Could you check a few things on this drawing? It's one solid part, dimensions in mm from its lowest x, y, z. A direction names the side the tool comes from. Coordinates: 2 decimals unless noted, no trailing zeros. Write each loop counter-clockwise with the first axis right and the second up, starting at its lowest first coordinate (ties: lowest second). Pieces come first, ordered by that corner, then holes. Notation, with made-up numbers: (45.25, 85.5) - (64.25, 85.5) arc R16 cw to (64.25, 93.5) - close; hole circle Ø7 at (56, -31.75). An arc over 180 degrees is marked (long way). Use one line per item in the form item = value. Start each with the question number.
(1) If we section it at B-B on y = 29.5: Please give me the cut outline in (x, z), then the cut area to 3 significant figures.
(2) If we section it at D-D on z = 19.25: Please give me the cut outline in (x, y).
(3) If we section it at A-A on x = 4: Please give me the cut outline in (y, z) (1 decimal).
(4) If I drill on probe 1 along Z at (x, y) = (14.5, 1); probe 2 along X at (y, z) = (13, 15.5) (1 decimal); probe 3 along X at (y, z) = (10, 20.25) (1 decimal), over which ranges is the centre line in solid material (lowest first)? Write a range as from..to.
(5) If we section it at C-C on z = 5: Please give me the cut outline in (x, y), then the cut area to 3 significant figures.
(6) For pin 1 Ø5 at (x, z) = (12, 14.5) entering from +Y; pin 2 Ø4 at (y, z) = (25.5, 5.5) entering from -X; pin 3 Ø12 at (y, z) = (9.5, 5) entering from -X; pin 4 Ø1.5 at (y, z) = (27, 3.5) entering from -X, each with a flat end and sliding along its axis, tell me the tip position at first contact or that it passes through.
(7) Thinking about a two-plate mould opening in Z: for the marked faces 3, 4 and 5, which applies, pulls with the +Z half, pulls with the -Z half, needs draft (parallel to the pull), parting line crosses it, or undercut?
(8) On a 3-axis mill with a long thin cutter (end or side, diameter ignored), from which of +Z, -Z, +X, -X, +Y, -Y can I reach the whole of each face in a straight line? I mean the marked faces 1 and 2. Say none if no direction works.
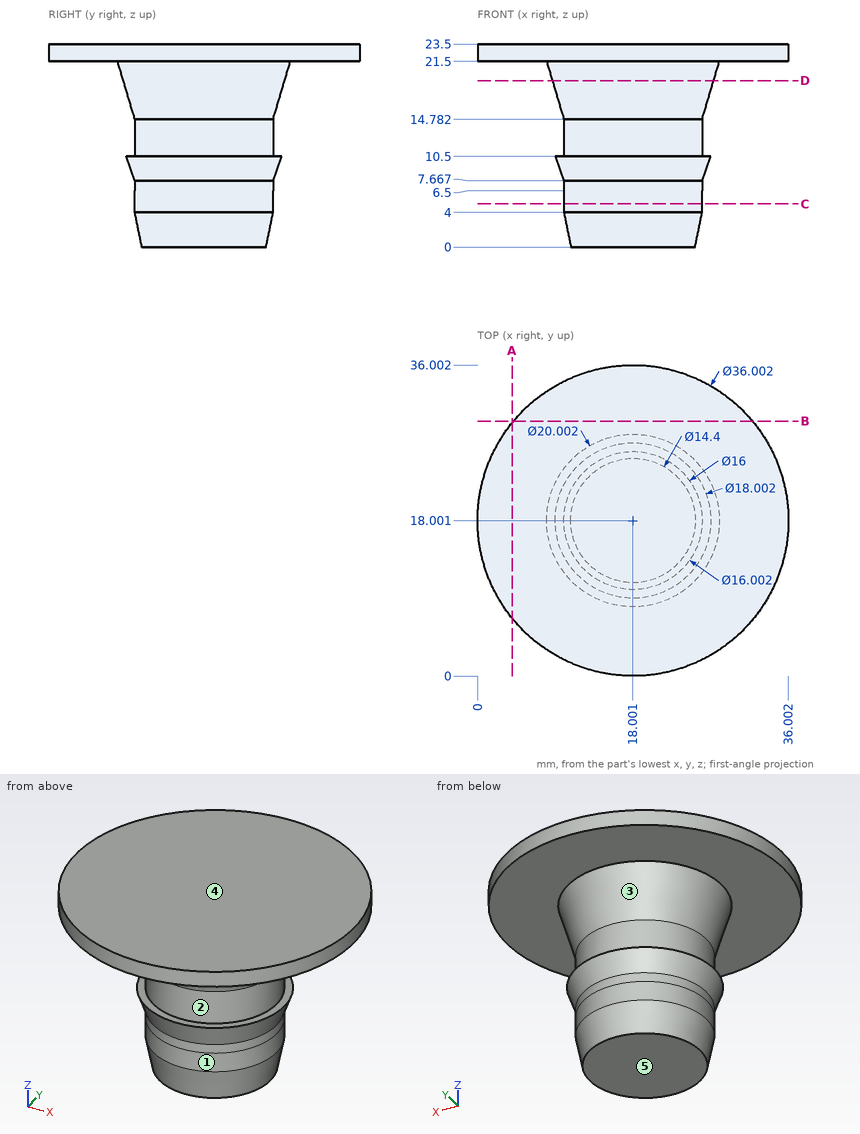
Reported:
q1.outline = (4.15, 21.5) - (31.85, 21.5) - (31.85, 23.5) - (4.15, 23.5) - close
q1.area = 55.4 mm2
q2.outline = circle Ø18.66 at (18, 18)
q3.outline = (6.7, 21.5) - (29.3, 21.5) - (29.3, 23.5) - (6.7, 23.5) - close
q4.probe_1 = 21.5..23.5
q4.probe_2 = 11.5..24.5
q4.probe_3 = 12.6..23.4
q5.outline = circle Ø16 at (18, 18)
q5.area = 201 mm2
q6.pin_1 = 25.35
q6.pin_2 = 12.19
q6.pin_3 = 10.4
q6.pin_4 = through
q7.face_3 = undercut
q7.face_4 = pulls with the +Z half
q7.face_5 = pulls with the -Z half
q8.face_1 = -Z
q8.face_2 = none
